Input: part model. Units: mm. Frame: model coordinates. A direction names the side the tool comes from. Round coordinates to 2 decimals unless told otherwise and drop trailing zeros. Loops run counter-clockwise (first coordinate to the right, second up) from the corner with the lowest first, then second, coordinate; pieces in that order, holes last. Notation, with made-up numbers: (70, 76) - (117, 76) arc R25 ccw to (117, 115) - close; hole circle Ø5 at (-17.5, 73). An arc over 180 degrees is marked (long way). Write each question's results on one line, items separated by ' | '.
from build123d import *

# Parameters (mm, degrees)
SKETCH1_W               = 70
SKETCH1_H               = 50
BOSS_EXTRUDE1_DEPTH     = 1.6383
SKETCH3_R               = 1.0795
CUT_EXTRUDE2_DEPTH      = 87.038851845
MIRROR2_COPY_1_SKETCH_R = 1.0795
MIRROR2_COPY_1_DEPTH    = 87.038851845
SKETCH4_W               = 6.35
SKETCH4_H               = 15.6718
SKETCH4_W_2             = 20.6756
SKETCH4_H_2             = 6.35
SKETCH4_W_3             = 5.5245
BOSS_EXTRUDE2_DEPTH     = 8.5344
SKETCH5_W               = 12.7
SKETCH5_H               = 15.9512
BOSS_EXTRUDE3_DEPTH     = 13.716
SKETCH7_W               = 49.276
SKETCH7_H               = 25.4
BOSS_EXTRUDE4_DEPTH     = 16.0655


with BuildPart() as part:
    # Sketch1 → Boss-Extrude1 (new body)
    with BuildSketch(Plane(origin=(0, 0, 0), x_dir=(1, 0, 0), z_dir=(0, 1, 0))):
        with Locations((35, 25)):
            Rectangle(SKETCH1_W, SKETCH1_H)
    extrude(amount=BOSS_EXTRUDE1_DEPTH)

    # Sketch3 → Cut-Extrude2 (cut, through all)
    with BuildSketch(Plane(origin=(0, 1.6383, 0), x_dir=(1, 0, 0), z_dir=(0, 1, 0))):
        with Locations(Location((2.0955, 2.0955, 0), (0, 0, 270))):
            Circle(SKETCH3_R)
    cut_extrude2 = extrude(amount=-CUT_EXTRUDE2_DEPTH, mode=Mode.SUBTRACT)

    # Mirror1: Cut-Extrude2 across plane
    add(cut_extrude2.mirror(Plane.XY.offset(-25)), mode=Mode.SUBTRACT)

    # Mirror2: Cut-Extrude2 across plane
    add(cut_extrude2.mirror(Plane(origin=(35, 0, 0), x_dir=(0, 0, 1), z_dir=(1, 0, 0))), mode=Mode.SUBTRACT)

    # Mirror2 copy 1 sketch → Mirror2 copy 1 (cut, through all)
    with BuildSketch(Plane(origin=(70, 1.6383, -50), x_dir=(-1, 0, 0), z_dir=(0, 1, 0))):
        with Locations(Location((2.0955, 2.0955, 0), (0, 0, 270))):
            Circle(MIRROR2_COPY_1_SKETCH_R)
    extrude(amount=-MIRROR2_COPY_1_DEPTH, mode=Mode.SUBTRACT)

    # Sketch4 → Boss-Extrude2 (add)
    with BuildSketch(Plane(origin=(0, 1.6383, 0), x_dir=(1, 0, 0), z_dir=(0, 1, 0))):
        with Locations((64.031, 15.1765)):
            Rectangle(SKETCH4_W, SKETCH4_H)
        with Locations((47.3559, 3.175)):
            Rectangle(SKETCH4_W_2, SKETCH4_H_2)
        with Locations((9.56945, 3.175)):
            Rectangle(SKETCH4_W_3, SKETCH4_H_2)
    extrude(amount=BOSS_EXTRUDE2_DEPTH)

    # Sketch5 → Boss-Extrude3 (add)
    with BuildSketch(Plane(origin=(0, 1.6383, 0), x_dir=(1, 0, 0), z_dir=(0, 1, 0))):
        with Locations((18.6817, 10.2616)):
            Rectangle(SKETCH5_W, SKETCH5_H)
    extrude(amount=BOSS_EXTRUDE3_DEPTH)

    # Sketch7 → Boss-Extrude4 (add)
    with BuildSketch(Plane(origin=(0, 1.6383, 0), x_dir=(1, 0, 0), z_dir=(0, 1, 0))):
        with Locations((31.75, 35.3696)):
            Rectangle(SKETCH7_W, SKETCH7_H)
    extrude(amount=BOSS_EXTRUDE4_DEPTH)


solid = part.part
1. Section query D-D, the plane x = 11.5. Output: boundary loops of the cut face in (y, z), plus the area to 3 significant figures.
Answer:
outline: (0, -50) - (1.64, -50) - (1.64, -48.07) - (17.7, -48.07) - (17.7, -22.67) - (1.64, -22.67) - (1.64, -6.35) - (10.17, -6.35) - (10.17, 0) - (0, 0) - close | area: 544 mm^2
2. Set-up query: faces 4 (the flat face through (25.032, 8, -10)), 5 (the flat face through (10, 6, -6.35)), 6 (the flat face through (47, 10.173, -3)). Return all of +Z, -Z, +X, -X, +Y, -Y with unobstructed straight access to the full face (end or side cutting, diameter ignored); none if empty.
Answer:
face 4: +Z, +Y | face 5: -X, +Y | face 6: +Z, +X, +Y
3. Section query B-B, the plane z = -4. Output: boundary loops of the cut face in (x, y), plus the area to 3 significant figures.
Answer:
outline: (0, 0) - (70, 0) - (70, 1.64) - (57.69, 1.64) - (57.69, 10.17) - (37.02, 10.17) - (37.02, 1.64) - (25.03, 1.64) - (25.03, 15.35) - (12.33, 15.35) - (12.33, 10.17) - (6.81, 10.17) - (6.81, 1.64) - (0, 1.64) - close | area: 512 mm^2
4. Contact query for flat-ended pins moving along their axis: pin 1 (1.8 mm diameter, centred on y = 6.5, z = -1.5, fed in from +X); pin 2 (4 mm diameter, centred on x = 16, z = -14, fed in from +Y); pin 3 (10 mm diameter, centred on y = 10.5, z = -19, fed in from -X). Output: stop coordinate, or through.
Answer:
pin 1: x = 57.69 | pin 2: y = 15.35 | pin 3: x = 7.11
5. Line query: line 1 (Z direction, x = 20.5, y = 14.5); line 2 (Z direction, x = 56, y = 8); line 3 (X direction, y = 9, z = -15.5). Output: solid intervals per line, ascending. Write a range as [from, to].
Answer:
line 1: [-48.07, -22.67], [-18.24, -2.29] | line 2: [-48.07, -22.67], [-6.35, 0] | line 3: [12.33, 25.03], [60.86, 67.21]
6. Section query C-C, the plane y = 12.25. Output: boundary loops of the cut face in (x, z), plus the area to 3 significant figures.
Answer:
outline: (7.11, -48.07) - (56.39, -48.07) - (56.39, -22.67) - (7.11, -22.67) - close; (12.33, -18.24) - (25.03, -18.24) - (25.03, -2.29) - (12.33, -2.29) - close | area: 1,450 mm^2
7. Section query A-A, the plane y = 4.5. Output: boundary loops of the cut face in (x, z), plus the area to 3 significant figures.
Answer:
outline: (6.81, -6.35) - (12.33, -6.35) - (12.33, -18.24) - (25.03, -18.24) - (25.03, -2.29) - (12.33, -2.29) - (12.33, 0) - (6.81, 0) - close; (7.11, -48.07) - (56.39, -48.07) - (56.39, -22.67) - (7.11, -22.67) - close; (37.02, -6.35) - (57.69, -6.35) - (57.69, 0) - (37.02, 0) - close; (60.86, -23.01) - (67.21, -23.01) - (67.21, -7.34) - (60.86, -7.34) - close | area: 1,720 mm^2
8. Mould query, pull axis Z, two halves, no side actions, for faces 1 (the flat face through (64, 6, -23.012)), 2 (the cylindrical face through (1.138, 0.831, -1.597)), 3 (the flat face through (10, 10.173, -3)). Classes: pulls with the +Z half, pulls with the -Z half, needs draft (parallel to the pull), parting line crosses it, or undercut.
Answer:
face 1: pulls with the -Z half | face 2: undercut | face 3: needs draft
